from build123d import *
from OCP.BRepFilletAPI import BRepFilletAPI_MakeFillet

# Parameters (mm, degrees)
SKETCH1_R           = 2.627
BOSS_EXTRUDE1_DEPTH = 6
BOSS_EXTRUDE2_START = -5.08
SKETCH1_3_W         = 38.1
SKETCH1_3_H         = 5.999999938
BOSS_EXTRUDE2_DEPTH = 22.86
SKETCH3_R           = 2.65
CUT_EXTRUDE1_DEPTH  = 44.260167546
FILLET1_R1          = 2.54
FILLET1_R2          = 5.08
SKETCH4_R           = 4.2145
SKETCH4_R_2         = 2.627
BOSS_EXTRUDE3_DEPTH = 1.5621
BOSS_EXTRUDE4_START = 8.5979
SKETCH4_2_R         = 4.2145
SKETCH4_2_R_2       = 2.627
BOSS_EXTRUDE4_DEPTH = 1.5621
CHAMFER2_SIZE       = 2.54


with BuildPart() as part:
    # Sketch1 → Boss-Extrude1 (new body)
    with BuildSketch(Plane(origin=(5.08, 0, 0), x_dir=(0, 0, -1), z_dir=(1, 0, 0))):
        Polygon((-19.05, 0), (-19.05, -10.16), (0, -25.4), (19.05, -10.16), (19.05, 0), align=None)
        with Locations((0, -16.51)):
            Circle(SKETCH1_R, mode=Mode.SUBTRACT)
    boss_extrude1 = extrude(amount=BOSS_EXTRUDE1_DEPTH)

    # Sketch1<3> → Boss-Extrude2 (add)
    with BuildSketch(Plane(origin=(5.08, 0, 0), x_dir=(0, 0, -1), z_dir=(1, 0, 0)).offset(BOSS_EXTRUDE2_START)):
        with Locations((0, 2.999999969)):
            Rectangle(SKETCH1_3_W, SKETCH1_3_H)
    boss_extrude2 = extrude(amount=BOSS_EXTRUDE2_DEPTH)

    # Sketch3 → Cut-Extrude1 (cut, through all)
    with BuildSketch(Plane(origin=(0, 5.999999938, 0), x_dir=(1, 0, 0), z_dir=(0, 1, 0))):
        with Locations(Location((16.51, 12.7, 0), (0, 0, 270))):
            Circle(SKETCH3_R)
        with Locations(Location((16.51, -12.7, 0), (0, 0, 90))):
            Circle(SKETCH3_R)
    cut_extrude1 = extrude(amount=-CUT_EXTRUDE1_DEPTH, mode=Mode.SUBTRACT)

    # Mirror2: Boss-Extrude2, Cut-Extrude1 across plane
    add(boss_extrude2.mirror(Plane(origin=(0, 0, 0), x_dir=(0, 0, 1), z_dir=(1, 0, 0))))
    add(cut_extrude1.mirror(Plane(origin=(0, 0, 0), x_dir=(0, 0, 1), z_dir=(1, 0, 0))), mode=Mode.SUBTRACT)

    # Mirror3: Boss-Extrude1 across plane
    add(boss_extrude1.mirror(Plane(origin=(0, 0, 0), x_dir=(0, 0, 1), z_dir=(1, 0, 0))))

    # Fillet1: one fillet with a radius per group of edges: ONE call of the kernel's fillet builder (fillet() takes one radius for all edges)
    fillet1_edges_1 = [part.edges().sort_by_distance(p)[0] for p in [
        (8.08, -10.16, 19.05),
        (8.08, -10.16, -19.05),
        (11.08, 0, 0),
        (22.86, 2.999999969, 19.05),
        (22.86, 2.999999969, -19.05),
        (-22.86, 2.999999969, -19.05),
        (-22.86, 2.999999969, 19.05),
        (-8.08, -10.16, -19.05),
        (-8.08, -10.16, 19.05),
        (-5.08, 0, 0),
        (-11.08, 0, 0),
        (5.08, 0, 0),
    ]]
    fillet1_edges_2 = [part.edges().sort_by_distance(p)[0] for p in [
        (8.08, -25.4, 0),
        (-8.08, -25.4, 0),
    ]]
    fillet1 = BRepFilletAPI_MakeFillet(part.part.solid().wrapped)
    for e in fillet1_edges_1:
        fillet1.Add(FILLET1_R1, e.wrapped)
    for e in fillet1_edges_2:
        fillet1.Add(FILLET1_R2, e.wrapped)
    add(Compound.cast(fillet1.Shape()), mode=Mode.REPLACE)

    # Sketch4 → Boss-Extrude3 (add)
    with BuildSketch(Plane.ZY.offset(-5.08)):
        with Locations(Location((0, -16.51, 0), (0, 0, 180))):
            Circle(SKETCH4_R)
        with Locations((0, -16.51)):
            Circle(SKETCH4_R_2, mode=Mode.SUBTRACT)
    extrude(amount=BOSS_EXTRUDE3_DEPTH)

    # Sketch4<2> → Boss-Extrude4 (add)
    with BuildSketch(Plane.ZY.offset(-5.08).offset(BOSS_EXTRUDE4_START)):
        with Locations(Location((0, -16.51, 0), (0, 0, 180))):
            Circle(SKETCH4_2_R)
        with Locations((0, -16.51)):
            Circle(SKETCH4_2_R_2, mode=Mode.SUBTRACT)
    extrude(amount=BOSS_EXTRUDE4_DEPTH)

    # Chamfer2
    # the kernel refuses this chamfer: 2.54 mm, written as the material it adds along each edge
    with BuildSketch(Plane(origin=(5.08, -16.51, 0), x_dir=(0, 0, -1), z_dir=(0, 1, 0))) as chamfer2_piece_1_section:
        Polygon((4.2145 + CHAMFER2_SIZE, 0), (4.2145, CHAMFER2_SIZE), (4.2145, 0), align=None)
    chamfer2_piece_1 = revolve(axis=Axis((5.08, -16.51, 0), (-1, 0, 0)), mode=Mode.PRIVATE)
    chamfer2_piece_1 = split(chamfer2_piece_1, bisect_by=Plane(origin=(3.5179, -16.51, 5.976913078), z_dir=(1, 0, 0)), keep=Keep.TOP, mode=Mode.PRIVATE)
    add(chamfer2_piece_1)
    with BuildSketch(Plane(origin=(-5.08, -16.51, 0), x_dir=(0, 0, -1), z_dir=(0, 1, 0))) as chamfer2_piece_2_section:
        Polygon((4.2145 + CHAMFER2_SIZE, 0), (4.2145, -CHAMFER2_SIZE), (4.2145, 0), align=None)
    chamfer2_piece_2 = revolve(axis=Axis((-5.08, -16.51, 0), (-1, 0, 0)), mode=Mode.PRIVATE)
    chamfer2_piece_2 = split(chamfer2_piece_2, bisect_by=Plane(origin=(-3.5179, -16.51, 5.976913078), z_dir=(-1, 0, 0)), keep=Keep.TOP, mode=Mode.PRIVATE)
    add(chamfer2_piece_2)


solid = part.part
The model under review builds one solid part; all positions refer to its coordinate system, in mm. A direction names the side the tool comes from. Round coordinates to 2 decimals unless told otherwise and drop trailing zeros. Write each loop counter-clockwise with the first axis right and the second up, starting at its lowest first coordinate (ties: lowest second). Pieces come first, ordered by that corner, then holes. Notation, with made-up numbers: M 59.25,86 L 76.25,86 A27 cw 76.25,114 Z; hole C 81.25,-38 d2. An arc over 180 degrees is marked long. Answer as CSV lines item,"result". Start each with the question number.
Q1. Tool access review of faces 4 (the face through (-18, 0, 0)), 5 (the face through (22.096, 3.042, 18.326)), 6 (the face through (4.316, -0.724, 0.267)): name each direction out of +Z, -Z, +X, -X, +Y, -Y from which nothing blocks a thin tool from reaching the whole face with its end or side.
Q2. Consider section A-A, the plane z = 12.7. Give the boundary of the cut face in (x, y), then the cut area to 3 significant figures.
Q3. Consider section B-B, the plane y = 2. Give the boundary of the cut face in (x, z), then the cut area to 3 significant figures.
Q4. Consider section C-C, the plane x = -16.51. Give the boundary of the cut face in (y, z), then the cut area to 3 significant figures.
Q5. Wall thickness on line 1 along X through (y, z) = (3.2, 12.7); line 2 along Y through (x, z) = (-6.9, 0); line 3 along X through (y, z) = (3.75, -11): over which ranges is each line inside the solid? List them lowest first.
Q6. Clearance check with flat-ended pins moving along their axes: P1, Ø5, axis at x = -16.51, z = -12.7, coming from the -Y side; P2, Ø2.5, axis at x = -1, z = -5, coming from the -Y side; P3, Ø17, axis at y = -15, z = 1, coming from the +X side; P4, Ø8.5, axis at x = -16.51, z = 12.7, coming from the -Y side. State where each tip first meets the part, or that it passes through.
Q7. Consider section D-D, the plane y = -16.51. Give the boundary of the cut face in (x, z), then the cut area to 3 significant figures.
Q8. The part is to be moulded in two halves that separate along Z. For faces 1 (the face through (-5.08, -8, 0)), 2 (the face through (0, 2, -19.05)), 3 (the face through (-18.861, 3.042, 11.477)), say which applies: +Z half, -Z half, draft (parallel to the pull), parting line (faces both ways), or undercut.
Result set:
1,face 4,"+Z, -Z, -X, -Y"
1,face 5,"+Z, +X, +Y, -Y"
1,face 6,"+Z, -Z"
2,outline,"M -22.86,0 L -19.16,0 L -19.16,6 L -22.86,6 Z; M -13.86,0 L -13.62,0 A2.54 cw -11.08,-2.54 L -11.08,-15.24 L -5.08,-15.24 L -5.08,-2.54 A2.54 cw -2.54,0 L 2.54,0 A2.54 cw 5.08,-2.54 L 5.08,-15.24 L 11.08,-15.24 L 11.08,-2.54 A2.54 cw 13.62,0 L 13.86,0 L 13.86,6 L -13.86,6 Z; M 19.16,0 L 22.86,0 L 22.86,6 L 19.16,6 Z"
2,area,"399 mm²"
3,outline,"M -22.86,-16.51 A2.54 ccw -20.32,-19.05 L 20.32,-19.05 A2.54 ccw 22.86,-16.51 L 22.86,16.51 A2.54 ccw 20.32,19.05 L -20.32,19.05 A2.54 ccw -22.86,16.51 Z; hole C -16.51,-12.7 d5.3; hole C -16.51,12.7 d5.3; hole C 16.51,-12.7 d5.3; hole C 16.51,12.7 d5.3"
3,area,"1,650 mm²"
4,outline,"M 0,-19.05 L 6,-19.05 L 6,-15.35 L 0,-15.35 Z; M 0,-10.05 L 6,-10.05 L 6,10.05 L 0,10.05 Z; M 0,15.35 L 6,15.35 L 6,19.05 L 0,19.05 Z"
4,area,"165 mm²"
5,line 1,"x = -22.86 to -19.16, -13.86 to 13.86, 19.16 to 22.86"
5,line 2,"y = -23.97 to -19.14, -13.88 to 6"
5,line 3,"x = -22.86 to -18.54, -14.48 to 14.48, 18.54 to 22.86"
6,P1,"passes through"
6,P2,"stops at y = 0"
6,P3,"stops at x = 11.08"
6,P4,"stops at y = -0.39"
7,outline,"M -11.08,-11.11 L -5.08,-11.11 L -5.08,-6.75 L -3.52,-5.19 L -3.52,-2.63 L -11.08,-2.63 Z; M -11.08,2.63 L -3.52,2.63 L -3.52,5.19 L -5.08,6.75 L -5.08,11.11 L -11.08,11.11 Z; M 3.52,-5.19 L 5.08,-6.75 L 5.08,-11.11 L 11.08,-11.11 L 11.08,-2.63 L 3.52,-2.63 Z; M 3.52,2.63 L 11.08,2.63 L 11.08,11.11 L 5.08,11.11 L 5.08,6.75 L 3.52,5.19 Z"
7,area,"225 mm²"
8,face 1,"draft"
8,face 2,"-Z half"
8,face 3,"undercut"
